from build123d import *

# Parameters (mm, degrees)
SKETCH_1_W      = 14.2
SKETCH_1_H      = 20
EXTRUDE_1_DEPTH = 7
SKETCH_1_3_W    = 5.8
SKETCH_1_3_H    = 6
SKETCH_1_3_R    = 1.5
EXTRUDE_2_DEPTH = 3
SKETCH_2_W      = 8
SKETCH_2_H      = 4
EXTRUDE_3_DEPTH = 2
SKETCH_3_R      = 1.028764089
EXTRUDE_4_DEPTH = 2
SKETCH_4_R      = 1.75
EXTRUDE_5_DEPTH = 20


with BuildPart() as part:
    # Sketch 1 → Extrude 1 (new body)
    with BuildSketch(Plane(origin=(0, 0, 0), x_dir=(1, 0, 0), z_dir=(0, 1, 0))):
        Rectangle(SKETCH_1_W, SKETCH_1_H)
    extrude(amount=EXTRUDE_1_DEPTH)

    # Sketch 1_3 → Extrude 2 (add)
    # profile 1 of 2: a face of its own
    with BuildSketch(Plane(origin=(0, 0, 0), x_dir=(1, 0, 0), z_dir=(0, 1, 0))):
        with Locations((-10, 7)):
            Rectangle(SKETCH_1_3_W, SKETCH_1_3_H)
        with Locations(Location((-10, 7, 0), (0, 0, 270))):
            Circle(SKETCH_1_3_R, mode=Mode.SUBTRACT)
    # profile 2 of 2: a face of its own
    with BuildSketch(Plane(origin=(0, 0, 0), x_dir=(1, 0, 0), z_dir=(0, 1, 0))):
        with Locations((10, 7)):
            Rectangle(SKETCH_1_3_W, SKETCH_1_3_H)
        with Locations(Location((10, 7, 0), (0, 0, 270))):
            Circle(SKETCH_1_3_R, mode=Mode.SUBTRACT)
    extrude(amount=EXTRUDE_2_DEPTH)

    # Sketch 2 → Extrude 3 (add)
    with BuildSketch(Plane(origin=(0, 7, 0), x_dir=(1, 0, 0), z_dir=(0, 1, 0))):
        with Locations((0, -7)):
            Rectangle(SKETCH_2_W, SKETCH_2_H)
    extrude(amount=EXTRUDE_3_DEPTH)

    # Sketch 3 → Extrude 4 (add)
    with BuildSketch(Plane(origin=(0, 7, 0), x_dir=(1, 0, 0), z_dir=(0, 1, 0))):
        with Locations(Location((4.398397856, 2.736092563, 0), (0, 0, 270))):
            Circle(SKETCH_3_R)
    extrude(amount=EXTRUDE_4_DEPTH)

    # Sketch 4 → Extrude 5 (add)
    with BuildSketch(Plane(origin=(0, 0, -10), x_dir=(-1, 0, 0), z_dir=(0, 0, -1))):
        with Locations((0, 3)):
            Circle(SKETCH_4_R)
    extrude(amount=EXTRUDE_5_DEPTH)


solid = part.part
Build history of the part. All positions in model axes, mm. A direction names the side the tool comes from. Round coordinates to 2 decimals unless told otherwise and drop trailing zeros. Order: outer loops, then holes, each group sorted by start corner. A loop starts at its lowest first (then second) coordinate and runs counter-clockwise, first axis right, second up. Notation, with made-up numbers: M 39,50.25 L 75,50.25 A27 ccw 75,66.25 Z; hole C 88,69.5 d3. An arc over 180 degrees is marked long. Use CSV: the item, a comma, the result in double quotes. Start each with the question number.
(1) Cut at C-C on y = 7.5. List the corners of the cut face in (x, z).
(2) Cut at B-B on z = -7. List the corners of the cut face in (x, y), then the cut area to 3 significant figures.
(3) Cut at A-A on x = -10. List the corners of the cut face in (y, z).
(4) Tool access for faces 1 (the face through (0.38, 1.29, -19.86)), 2 (the face through (8.7, 3, -8.4)), 3 (the face through (-4, 8, 7)), 4 (the face through (-10, 1, -4)): list every direction of +Z, -Z, +X, -X, +Y, -Y with a clear straight run to the whole face (end or side of a thin tool).
(5) Mould opens along Z. For faces 5 (the face through (4, 9, -3)), 6 (the face through (0, 8, 9)), 7 (the face through (9.1, 1.5, -8.2)) say: +Z half, -Z half, draft (parallel to the pull), parting line (faces both ways), or undercut.
(6) Flat gauge pins, fed straight in: P1, Ø1.6, axis at x = -1, y = 8.5, coming from the +Z side; P2, Ø2.5, axis at x = -9, y = 1.5, coming from the +Z side; P3, Ø10, axis at x = 3.5, z = -16, coming from the -Y side; P4, Ø2.5, axis at x = -10, z = -7, coming from the -Y side. Where does each tip first touch, or does it go through?
(7) Drill centre lines: probe 1 along X at (y, z) = (1.75, -7); probe 2 along X at (y, z) = (4, -7); probe 3 along Y at (x, z) = (2.25, 3). Where is each one in solid material? Low to high.
(8) Cut at D-D on x = 0. List the corners of the cut face in (y, z), then the cut area to 3 significant figures.
Findings:
1,outline,"M -4,5 L 4,5 L 4,9 L -4,9 Z; C 4.4,-2.74 d2.06"
2,outline,"M -12.9,0 L -11.5,0 L -11.5,3 L -12.9,3 Z; M -8.5,0 L 8.5,0 L 8.5,3 L 7.1,3 L 7.1,7 L -7.1,7 L -7.1,3 L -8.5,3 Z; M 11.5,0 L 12.9,0 L 12.9,3 L 11.5,3 Z"
2,area,"116 mm^2"
3,outline,"M 0,-10 L 3,-10 L 3,-8.5 L 0,-8.5 Z; M 0,-5.5 L 3,-5.5 L 3,-4 L 0,-4 Z"
4,face 1,"-Z"
4,face 2,"+Z, -Z, +X, +Y"
4,face 3,"+Z, -Z, -X, +Y"
4,face 4,"+Z, -X, +Y, -Y"
5,face 5,"draft"
5,face 6,"+Z half"
5,face 7,"undercut"
6,P1,"stops at z = 9"
6,P2,"stops at z = -4"
6,P3,"stops at y = 1.25"
6,P4,"passes through"
7,probe 1,"x = -12.9 to -11.5, -8.5 to 8.5, 11.5 to 12.9"
7,probe 2,"x = -7.1 to 7.1"
7,probe 3,"y = 0 to 7"
8,outline,"M 0,-10 L 1.25,-10 L 1.25,-30 L 4.75,-30 L 4.75,-10 L 7,-10 L 7,5 L 9,5 L 9,9 L 7,9 L 7,10 L 0,10 Z"
8,area,"218 mm^2"
